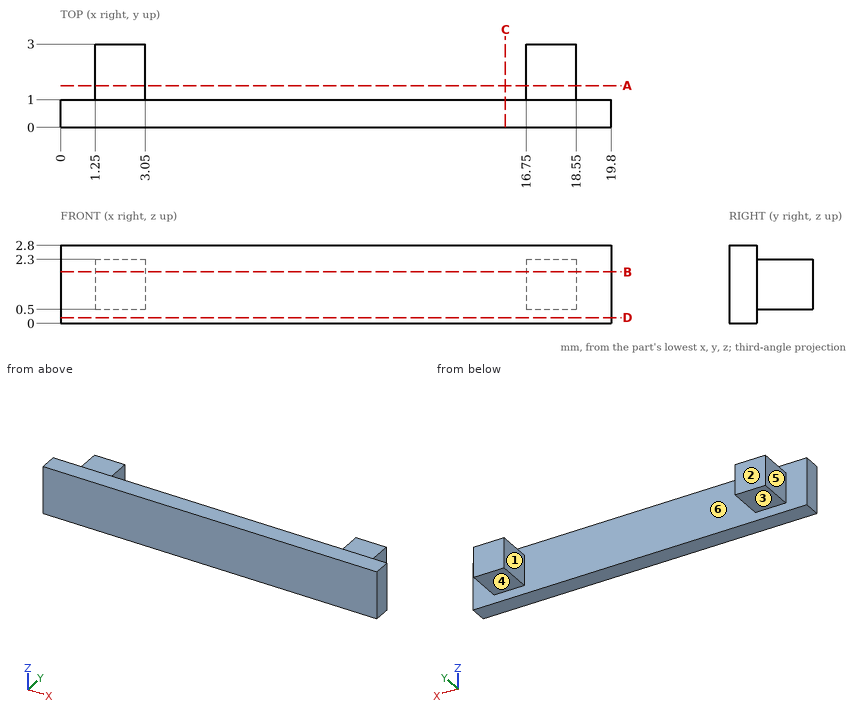
Geometry: see drawing. Coordinates: mm, zero at the bounding-box minimum. A direction names the side the tool comes from. Round coordinates to 2 decimals unless told otherwise and drop trailing zeros. Loops run counter-clockwise (first coordinate to the right, second up) from the corner with the lowest first, then second, coordinate; pieces in that order, holes last. Notation, with made-up numbers: (34, 55.5) - (85, 55.5) arc R24 ccw to (85, 87.5) - close; hole circle Ø11 at (4, 6.5). An arc over 180 degrees is marked (long way). Write item = value, one per line. Start each with the question number.
(1) Set-up query: the marked faces 1, 2 and 3. Return all of +Z, -Z, +X, -X, +Y, -Y with unobstructed straight access to the full face (end or side cutting, diameter ignored); none if empty.
(2) Pin query (flat end, axial travel): pin 1 (1.4 mm diameter, centred on y = 2, z = 1, fed in from -X); pin 2 (0.9 mm diameter, centred on x = 2, y = 2, fed in from +Z); pin 3 (0.9 mm diameter, centred on x = 2.5, y = 2, fed in from -Z). Return the tip coordinate at first contact, or that it passes through.
(3) Section query D-D, the plane z = 0.2. Output: boundary loops of the cut face in (x, y), plus the area to 3 significant figures.
(4) Section query B-B, the plane z = 1.85. Output: boundary loops of the cut face in (x, y).
(5) Section query C-C, the plane x = 16. Output: boundary loops of the cut face in (y, z), plus the area to 3 significant figures.
(6) Pull-direction query (X, two-part tool) for the marked faces 4, 5 and 6; classes: +X half, -X half, draft (parallel to the pull), parting line (faces both ways), or undercut.
(7) Ray query, line 1 along X through (y, z) = (2.15, 2.1); line 2 along Y through (x, z) = (15.5, 0.85); line 3 along Z through (x, y) = (18, 1.8). Return the intervals inside material, ascending. Write a range as from..to.
(8) Section query A-A, the plane y = 1.5. Output: boundary loops of the cut face in (x, z), plus the area to 3 significant figures.
Conclusion:
q1.face_1 = +Z, -Z, +Y
q1.face_2 = +Z, -Z, +X, -X, +Y
q1.face_3 = -Z, +X, -X, +Y
q2.pin_1 = 1.25
q2.pin_2 = 2.3
q2.pin_3 = 0.5
q3.outline = (0, 0) - (19.8, 0) - (19.8, 1) - (0, 1) - close
q3.area = 19.8 mm2
q4.outline = (0, 0) - (19.8, 0) - (19.8, 1) - (18.55, 1) - (18.55, 3) - (16.75, 3) - (16.75, 1) - (3.05, 1) - (3.05, 3) - (1.25, 3) - (1.25, 1) - (0, 1) - close
q5.outline = (0, 0) - (1, 0) - (1, 2.8) - (0, 2.8) - close
q5.area = 2.80 mm2
q6.face_4 = draft
q6.face_5 = -X half
q6.face_6 = undercut
q7.line_1 = 1.25..3.05, 16.75..18.55
q7.line_2 = 0..1
q7.line_3 = 0.5..2.3
q8.outline = (1.25, 0.5) - (3.05, 0.5) - (3.05, 2.3) - (1.25, 2.3) - close; (16.75, 0.5) - (18.55, 0.5) - (18.55, 2.3) - (16.75, 2.3) - close
q8.area = 6.48 mm2
